Input: part model. Units: mm. Frame: model coordinates. A direction names the side the tool comes from. Coordinates: 2 decimals unless noted, no trailing zeros. Order: outer loops, then holes, each group sorted by start corner. A loop starts at its lowest first (then second) coordinate and runs counter-clockwise, first axis right, second up. Notation, with made-up numbers: (57, 12.5) - (91, 12.5) arc R24 cw to (91, 31.5) - close; hole circle Ø1 at (6, 51). An arc over 180 degrees is marked (long way). One line per question, with ' | ' between items.
from build123d import *

# Parameters (mm, degrees)
SKETCH_W        = 18
SKETCH_H        = 5
PAD_DEPTH       = 4
PAD_TAPER       = 23
PAD_FACE5_W     = 5
PAD_FACE5_H     = 18
PAD001_DEPTH    = 10.5
SKETCH001_W     = 16.5
SKETCH001_H     = 3.5
POCKET_DEPTH    = 10.5
SKETCH002_W     = 16.5
SKETCH002_H     = 3.5
POCKET001_DEPTH = 3
POCKET001_TAPER = 22
SKETCH003_W     = 18.711727
SKETCH003_H     = 3.5
POCKET002_DEPTH = 2


with BuildPart() as part:
    # Sketch → Pad (new body)
    with BuildSketch(Plane.XY):
        Rectangle(SKETCH_W, SKETCH_H)
    extrude(amount=PAD_DEPTH, taper=PAD_TAPER)

    # Pad Face5 → Pad001 (add)
    with BuildSketch(Plane(origin=(0, 0, 0), x_dir=(0, -1, 0), z_dir=(0, 0, -1))):
        Rectangle(PAD_FACE5_W, PAD_FACE5_H)
    extrude(amount=PAD001_DEPTH)

    # Sketch001 (on Face8 of Pad001) → Pocket (cut)
    with BuildSketch(Plane(origin=(0, 0, -10.5), x_dir=(1, 0, 0), z_dir=(0, 0, -1))):
        Rectangle(SKETCH001_W, SKETCH001_H)
    extrude(amount=-POCKET_DEPTH, mode=Mode.SUBTRACT)

    # Sketch002 (on Face15 of Pocket) → Pocket001 (cut)
    with BuildSketch(Plane(origin=(0, 0, 0), x_dir=(1, 0, 0), z_dir=(0, 0, -1))):
        Rectangle(SKETCH002_W, SKETCH002_H)
    extrude(amount=-POCKET001_DEPTH, taper=POCKET001_TAPER, mode=Mode.SUBTRACT)

    # Sketch003 (on Face8 of Pocket001) → Pocket002 (cut)
    with BuildSketch(Plane(origin=(0, 0, -10.5), x_dir=(1, 0, 0), z_dir=(0, 0, -1))):
        with Locations((0.078186, 0)):
            Rectangle(SKETCH003_W, SKETCH003_H)
    extrude(amount=-POCKET002_DEPTH, mode=Mode.SUBTRACT)


solid = part.part
Item 1: Ray query, line 1 (Y direction, x = 6.75, z = -8.5); line 2 (Z direction, x = 2.5, y = -0.3); line 3 (Y direction, x = -5, z = 2). Return the intervals inside material, ascending.
Data:
line 1: -2.5 to -1.75, 1.75 to 2.5 | line 2: 3 to 4 | line 3: -1.65 to -0.94, 0.94 to 1.65
Item 2: Access query for faces 5 (the face through (0, -2.5, -5)), 6 (the face through (0, 0, 3)). Directions: +Z, -Z, +X, -X, +Y, -Y. A direction counts if a zero-diameter tool reaches every point of the face in a straight line with its end or side. Return the directions, or none.
Data:
face 5: +Z, -Z, +X, -X, -Y | face 6: -Z
Item 3: Section A-A on z = -4.75. Return the cut outline in (x, y).
Data:
outline: (-9, -2.5) - (9, -2.5) - (9, 2.5) - (-9, 2.5) - close; hole (-8.25, -1.75) - (8.25, -1.75) - (8.25, 1.75) - (-8.25, 1.75) - close
Item 4: Draft query along Y for faces 1 (the face through (0, 2.5, -5)), 2 (the face through (8.25, 0, -4)), 3 (the face through (0, 0, 4)), 4 (the face through (0, -1.75, -5)). Return one class per face: released by +Y, released by -Y, zero draft, split by the parting line, or undercut.
Data:
face 1: released by +Y | face 2: undercut | face 3: zero draft | face 4: undercut
Item 5: Contact query for a flat-ended pin moving along its axis: P1, Ø0.5, axis at x = 2.5, y = 0.5, coming from the -Z side. Output: stop coordinate, or through.
Data:
P1: z = 2.48
